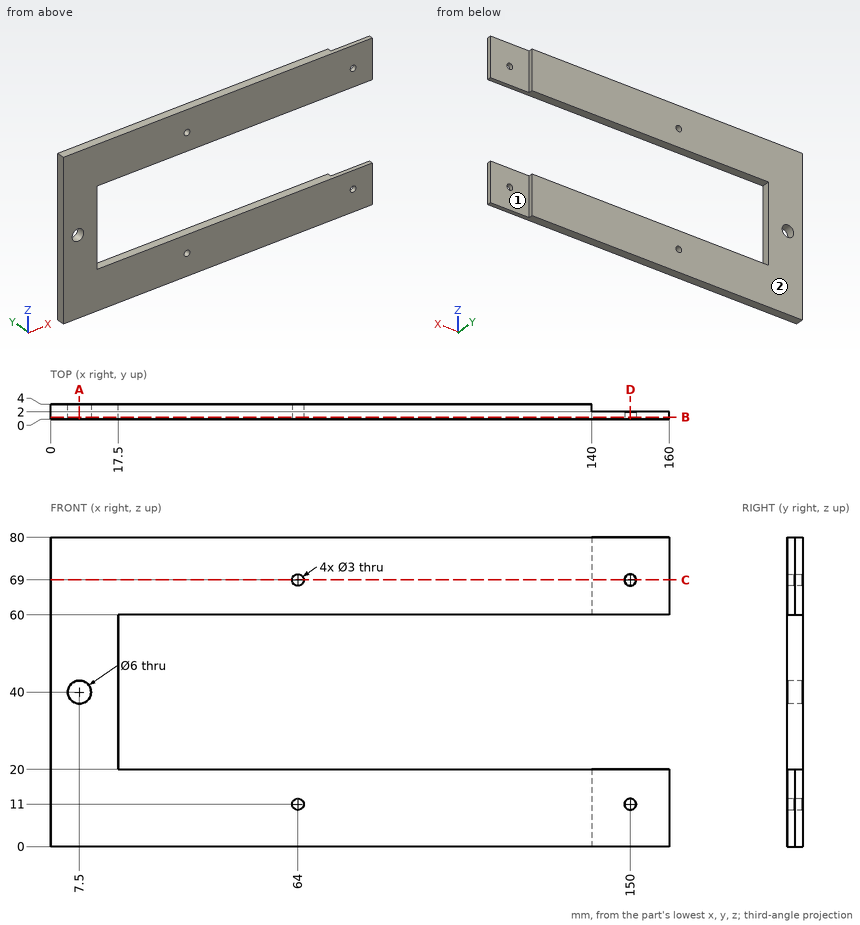
The figure shows three views and two pictorial views of one solid part (mm, origin at its lowest corner). Answer the questions. A direction names the side the tool comes from. Coordinates: 2 decimals unless noted, no trailing zeros. Loops run counter-clockwise (first coordinate to the right, second up) from the corner with the lowest first, then second, coordinate; pieces in that order, holes last. Notation, with made-up numbers: (28, 83.25) -> (39, 83.25) arc R19 ccw to (39, 112.25) -> close; hole circle Ø1 at (-5, 88). An arc over 180 degrees is marked (long way). Use one line per item in the form item = value. Start each with the question number.
Item 1: Flat-ended cylindrical pins translate along their axes: pin 1 Ø22 at (x, z) = (154, 72) entering from +Y; pin 2 Ø0.6 at (y, z) = (2.5, 8.5) entering from +X; pin 3 Ø2 at (y, z) = (0.5, 40) entering from +X. Find the tip coordinate at first contact, or state that the pin passes through.
Item 2: Consider L1, parallel to X at y = 1.4, z = 69; L2, parallel to Z at x = 150, y = 0.7; L3, parallel to Z at x = 84, y = 1.75. Determine where each line is inside the solid, lowest interval first. Write a range as [from, to].
Item 3: The part is cut by section B-B on y = 0.6. Determine the outline of the cut face in (x, z).
Item 4: A tool of negligible diameter and unlimited length cuts with its end or side. For the marked faces 1 and 2, from which of +Z, -Z, +X, -X, +Y, -Y can it reach the whole face along a straight path? Write none if from no direction.
Item 5: The part is cut by section A-A on x = 7.5. Determine the outline of the cut face in (y, z), then the cut area to 3 significant figures.
Item 6: The part is cut by section C-C on z = 69. Determine the outline of the cut face in (x, y), then the cut area to 3 significant figures.
Item 7: The part is cut by section D-D on x = 150. Determine the outline of the cut face in (y, z), then the cut area to 3 significant figures.
Answer key:
q1.pin_1 = 2
q1.pin_2 = 140
q1.pin_3 = 17.5
q2.L1 = [0, 62.5], [65.5, 148.5], [151.5, 160]
q2.L2 = [0, 9.5], [12.5, 20], [60, 67.5], [70.5, 80]
q2.L3 = [0, 20], [60, 80]
q3.outline = (0, 0) -> (160, 0) -> (160, 20) -> (17.5, 20) -> (17.5, 60) -> (160, 60) -> (160, 80) -> (0, 80) -> close; hole circle Ø6 at (7.5, 40); hole circle Ø3 at (64, 11); hole circle Ø3 at (64, 69); hole circle Ø3 at (150, 11); hole circle Ø3 at (150, 69)
q4.face_1 = +Z, -Z, +X, +Y
q4.face_2 = +Z, -Z, +X, -X, +Y
q5.outline = (0, 0) -> (4, 0) -> (4, 37) -> (0, 37) -> close; (0, 43) -> (4, 43) -> (4, 80) -> (0, 80) -> close
q5.area = 296 mm2
q6.outline = (0, 0) -> (62.5, 0) -> (62.5, 4) -> (0, 4) -> close; (65.5, 0) -> (148.5, 0) -> (148.5, 2) -> (140, 2) -> (140, 4) -> (65.5, 4) -> close; (151.5, 0) -> (160, 0) -> (160, 2) -> (151.5, 2) -> close
q6.area = 582 mm2
q7.outline = (0, 0) -> (2, 0) -> (2, 9.5) -> (0, 9.5) -> close; (0, 12.5) -> (2, 12.5) -> (2, 20) -> (0, 20) -> close; (0, 60) -> (2, 60) -> (2, 67.5) -> (0, 67.5) -> close; (0, 70.5) -> (2, 70.5) -> (2, 80) -> (0, 80) -> close
q7.area = 68.0 mm2
